Input: part model. Units: mm. Frame: model coordinates. A direction names the side the tool comes from. Coordinates: 2 decimals unless noted, no trailing zeros. Order: outer loops, then holes, each group sorted by start corner. A loop starts at its lowest first (then second) coordinate and runs counter-clockwise, first axis right, second up. Notation, with made-up numbers: (57, 39.5) -> (110, 39.5) arc R15 ccw to (110, 60.5) -> close; hole circle Ø11 at (11, 60.5). An arc over 180 degrees is marked (long way). Answer as CSV lines item,"result".
from build123d import *

# Parameters (mm, degrees)
SKETCH_1_R          = 1.9
EXTRUDE_1_DEPTH     = 0.5
SKETCH_2_R          = 1.7
EXTRUDE_2_DEPTH     = 2.9
SKETCH_3_R          = 1
EXTRUDE_3_DEPTH     = 2.6
SKETCH_4_W          = 0.5
SKETCH_4_H          = 25.5
SKETCH_4_H_2        = 27
SKETCH_4_W_2        = 0.7
SKETCH_4_H_3        = 0.791326506
EXTRUDE_4_DEPTH     = 0.25
CUT_EXTRUDE_2_REACH = 29.133
SKETCH_5_W          = 6.962557402
SKETCH_5_H          = 5.683720328
SKETCH_5_W_2        = 5.258758642
SKETCH_5_H_2        = 3


with BuildPart() as part:
    # Эскиз1 → Бобышка-Вытянуть1 (new body)
    with BuildSketch(Plane(origin=(0, 0, 0), x_dir=(1, 0, 0), z_dir=(0, 1, 0))):
        with Locations(Location((0, 0, 0), (0, 0, 270))):
            Circle(SKETCH_1_R)
    extrude(amount=EXTRUDE_1_DEPTH)

    # Эскиз2 → Бобышка-Вытянуть2 (add)
    with BuildSketch(Plane(origin=(0, 0.5, 0), x_dir=(1, 0, 0), z_dir=(0, 1, 0))):
        with Locations(Location((0, 0, 0), (0, 0, 270))):
            Circle(SKETCH_2_R)
    extrude(amount=EXTRUDE_2_DEPTH)

    # Эскиз3 → Бобышка-Вытянуть3 (add)
    with BuildSketch(Plane(origin=(0, 3.4, 0), x_dir=(1, 0, 0), z_dir=(0, 1, 0))):
        with Locations(Location((0, 0, 0), (0, 0, 270))):
            Circle(SKETCH_3_R)
    extrude(amount=EXTRUDE_3_DEPTH)

    # Эскиз4 → Бобышка-Вытянуть4 (add, symmetric)
    with BuildSketch(Plane.XY):
        with Locations((1.27, -12.75)):
            Rectangle(SKETCH_4_W, SKETCH_4_H)
        with Locations((-1.27, -13.5)):
            Rectangle(SKETCH_4_W, SKETCH_4_H_2)
        with Locations((1.27, -3.489413043)):
            Rectangle(SKETCH_4_W_2, SKETCH_4_H_3)
        with Locations((-1.27, -3.489413043)):
            Rectangle(SKETCH_4_W_2, SKETCH_4_H_3)
    extrude(amount=EXTRUDE_4_DEPTH, both=True)

    # Вырез-Вытянуть2: up to this face of the body (flat: up to its plane)
    cut_extrude_2_end = Plane(part.part.faces().sort_by_distance((0, 6, 0))[0])
    # Эскиз5 → Вырез-Вытянуть2 (cut, up to the picked face)
    with BuildSketch(Plane.XZ, mode=Mode.PRIVATE) as cut_extrude_2_sk1:
        Rectangle(SKETCH_5_W, SKETCH_5_H)
        Rectangle(SKETCH_5_W_2, SKETCH_5_H_2, mode=Mode.SUBTRACT)
    cut_extrude_2_tool1 = split(extrude(cut_extrude_2_sk1.sketch, amount=-CUT_EXTRUDE_2_REACH, mode=Mode.PRIVATE), bisect_by=cut_extrude_2_end, keep=Keep.BOTH, mode=Mode.PRIVATE)
    add(cut_extrude_2_tool1.solids().sort_by(Axis((0, 0, -2.751981), (0, 1, 0)))[0], mode=Mode.SUBTRACT)


solid = part.part
1. Cut plane B-B (x = 0). Return the cut outline in (y, z), plus the area to 3 significant figures.
Findings:
outline,"(0, -1.5) -> (3.4, -1.5) -> (3.4, -1) -> (6, -1) -> (6, 1) -> (3.4, 1) -> (3.4, 1.5) -> (0, 1.5) -> close"
area,"15.4 mm2"
2. Cut plane A-A (y = -8.5). Return the cut outline in (x, z), plus the area to 3 significant figures.
Findings:
outline,"(-1.52, -0.25) -> (-1.02, -0.25) -> (-1.02, 0.25) -> (-1.52, 0.25) -> close; (1.02, -0.25) -> (1.52, -0.25) -> (1.52, 0.25) -> (1.02, 0.25) -> close"
area,"0.500 mm2"
3. Reachability of faces 1 (the face through (-1.7, 1.9, 0)), 2 (the face through (1, 3.4, -1)), 3 (the face through (1.7, 1.9, 0)) from +Z, -Z, +X, -X, +Y, -Y: full face, straight path, thin tool, end or side. Return the list, or none.
Findings:
face 1,"-X, +Y"
face 2,"+Y"
face 3,"+X, +Y"
4. Cut plane C-C (z = 0.6). Return the cut outline in (x, y), plus the area to 3 significant figures.
Findings:
outline,"(-1.8, 0) -> (1.8, 0) -> (1.8, 0.5) -> (1.59, 0.5) -> (1.59, 3.4) -> (0.8, 3.4) -> (0.8, 6) -> (-0.8, 6) -> (-0.8, 3.4) -> (-1.59, 3.4) -> (-1.59, 0.5) -> (-1.8, 0.5) -> close"
area,"15.2 mm2"
5. Ray query, line 1 along X through (y, z) = (-24, 0.05); line 2 along Y through (x, z) = (-0.3, -0.1); line 3 along Y through (x, z) = (-1.3, -1.05). Return the intervals inside material, ascending.
Findings:
line 1,"x = -1.52 to -1.02, 1.02 to 1.52"
line 2,"y = 0 to 6"
line 3,"y = 0 to 3.4"
6. Contact query for flat-ended pins moving along their axis: pin 1 (0.9 mm diameter, centred on x = -0.5, z = 0.5, fed in from -Y); pin 2 (0.6 mm diameter, centred on y = -1.5, z = 0, fed in from -X); pin 3 (2 mm diameter, centred on x = -0.5, y = -4.5, fed in from -Z). Output: stop coordinate, or through.
Findings:
pin 1,"stops at y = 0"
pin 2,"stops at x = -1.52"
pin 3,"stops at z = -0.25"
